from build123d import *

# Parameters (mm, degrees)
BOSS_EXTRUDE1_DEPTH = 3.048
SKETCH2_R           = 1.355900406
CUT_EXTRUDE1_DEPTH  = 430.898988368
SKETCH3_R           = 1.524
CUT_EXTRUDE2_DEPTH  = 430.898988368
CUT_EXTRUDE3_DEPTH  = 430.898988368
BOSS_EXTRUDE2_DEPTH = 3.048
SKETCH5_W           = 73.1256
SKETCH5_H           = 52.8987
SKETCH5_W_2         = 9.017
SKETCH5_H_2         = 13.74935
CUT_EXTRUDE4_DEPTH  = 430.898988368


with BuildPart() as part:
    # Sketch1 → Boss-Extrude1 (new body)
    with BuildSketch(Plane.XY):
        with BuildLine():
            Line((-309.8086, 128.8851), (-305.87795, 128.8851))
            Line((-305.87795, 128.8851), (-301.9473, 132.81575))
            Line((-301.9473, 132.81575), (-301.9473, 150.9704))
            ThreePointArc((-301.9473, 150.9704), (-303.063223164, 153.664476836), (-305.7573, 154.7804))
            Line((-305.7573, 154.7804), (-397.247125, 154.7804))
            ThreePointArc((-397.247125, 154.7804), (-399.946077222, 153.659592612), (-401.0571, 150.956597849))
            Line((-401.0571, 150.956597849), (-401.0571, 148.341))
            Line((-401.0571, 148.341), (-399.1521, 148.341))
            Line((-399.1521, 148.341), (-399.1521, 95.6449))
            Line((-399.1521, 95.6449), (-401.0571, 95.6449))
            Line((-401.0571, 95.6449), (-401.0571, 91.659304166))
            ThreePointArc((-401.0571, 91.659304166), (-399.951018769, 88.947400452), (-397.2472, 87.8217))
            Line((-397.2472, 87.8217), (-378.5565, 87.8217))
            Line((-378.5565, 87.8217), (-368.3165, 91.1883))
            Line((-368.3165, 91.1883), (-315.9973, 91.1883))
            Line((-315.9973, 91.1883), (-305.7573, 87.8217))
            ThreePointArc((-305.7573, 87.8217), (-303.063223164, 88.937623164), (-301.9473, 91.6317))
            Line((-301.9473, 91.6317), (-301.9473, 111.74645))
            Line((-301.9473, 111.74645), (-305.87795, 115.6771))
            Line((-305.87795, 115.6771), (-309.8086, 115.6771))
            Line((-309.8086, 115.6771), (-314.0123, 115.6771))
            Line((-314.0123, 115.6771), (-314.0123, 128.8851))
            Line((-314.0123, 128.8851), (-309.8086, 128.8851))
        make_face()
        Polygon((-395.3675, 92.9525), (-395.3675, 149.2432), (-309.8086, 149.2432), (-309.8086, 132.81575), (-318.2033, 132.81575), (-318.2033, 111.74645), (-309.8086, 111.74645), (-309.8086, 92.9525), align=None, mode=Mode.SUBTRACT)
    extrude(amount=BOSS_EXTRUDE1_DEPTH)

    # Sketch2 → Cut-Extrude1 (cut, through all)
    with BuildSketch(Plane(origin=(0, 0, 0), x_dir=(-1, 0, 0), z_dir=(0, 0, -1))):
        with Locations((305.7573, 150.9704)):
            Circle(SKETCH2_R)
        with Locations((397.247125, 150.9704)):
            Circle(SKETCH2_R)
        with Locations((397.2472, 91.6317)):
            Circle(SKETCH2_R)
        with Locations((305.7573, 91.6317)):
            Circle(SKETCH2_R)
    extrude(amount=-CUT_EXTRUDE1_DEPTH, mode=Mode.SUBTRACT)

    # Sketch3 → Cut-Extrude2 (cut, through all)
    with BuildSketch(Plane(origin=(0, 0, 0), x_dir=(-1, 0, 0), z_dir=(0, 0, -1))):
        with Locations((305.7573, 150.9704)):
            Circle(SKETCH3_R)
        with Locations((397.247125, 150.9704)):
            Circle(SKETCH3_R)
        with Locations((397.2472, 91.6317)):
            Circle(SKETCH3_R)
        with Locations((305.7573, 91.6317)):
            Circle(SKETCH3_R)
    extrude(amount=-CUT_EXTRUDE2_DEPTH, mode=Mode.SUBTRACT)

    # Sketch4 → Cut-Extrude3 (cut, through all)
    with BuildSketch(Plane.XY.offset(3.048)):
        Polygon((-301.9473, 133.57775), (-305.87795, 129.6471), (-314.0123, 129.6471), (-314.0123, 113.6451), (-305.87795, 113.6451), (-301.9473, 109.71445), align=None)
    extrude(amount=-CUT_EXTRUDE3_DEPTH, mode=Mode.SUBTRACT)

    # Sketch4<4> → Boss-Extrude2 (add)
    with BuildSketch(Plane.XY.offset(3.048)):
        Polygon((-318.2033, 111.74645), (-318.2033, 132.81575), (-309.8086, 132.81575), (-309.8086, 149.2432), (-395.3675, 149.2432), (-395.3675, 92.9525), (-309.8086, 92.9525), (-309.8086, 111.74645), align=None)
    extrude(amount=-BOSS_EXTRUDE2_DEPTH)

    # Sketch5 → Cut-Extrude4 (cut, through all)
    with BuildSketch(Plane.XY.offset(3.048)):
        with Locations((-357.6871, 121.98105)):
            Rectangle(SKETCH5_W, SKETCH5_H)
        with Locations((-316.6158, 141.555725)):
            Rectangle(SKETCH5_W_2, SKETCH5_H_2)
        with Locations((-316.6158, 102.406375)):
            Rectangle(SKETCH5_W_2, SKETCH5_H_2)
    extrude(amount=-CUT_EXTRUDE4_DEPTH, mode=Mode.SUBTRACT)


solid = part.part
Verification items for the finished model (mm, model axes). A direction names the side the tool comes from. Coordinates: 2 decimals unless noted, no trailing zeros. Write each loop counter-clockwise with the first axis right and the second up, starting at its lowest first coordinate (ties: lowest second). Pieces come first, ordered by that corner, then holes. Notation, with made-up numbers: M 8,45 L 49,45 A18 cw 49,50 Z; hole C -38.75,3 d6. An arc over 180 degrees is marked long. Use CSV: the item, a comma, the result in double quotes.
Q1. Set-up check for faces 4 (the flat face through (-303.885, 131.64, 1.545)), 5 (the flat face through (-310.95, 89.53, 1.5)), 6 (the flat face through (-317, 134.681, 2)), 7 (the flat face through (-400, 95.645, 2)): record each of +Z, -Z, +X, -X, +Y, -Y from which the full face is reachable in a straight line by a thin tool's end or side.
Computed values:
face 4,"+Z, -Z, +X"
face 5,"+Z, -Z, -Y"
face 6,"+Z, -Z"
face 7,"+Z, -Z, -X"
Q2. Section check C-C, the plane z = 0.7. State how many separate pieces and enclosed holes the cut face has, and give its area (3 significant figures).
Computed values:
separate pieces,"1"
enclosed holes,"5"
area,"1,960 mm²"
Q3. Thickness scan on line 1 along Y through (x, z) = (-317, 1.6); line 2 along Y through (x, z) = (-365, 2); line 3 along X through (y, z) = (105, 0.35). Record the ranges inside material, lowest first. Write a range as [from, to].
Computed values:
line 1,"[91.19, 95.53], [109.28, 134.68], [148.43, 154.78]"
line 2,"[91.19, 95.53], [148.43, 154.78]"
line 3,"[-399.15, -394.25], [-312.11, -301.95]"
Q4. Go/stop test with flat-tipped pins: P1, Ø1.5, axis at y = 144.5, z = 2, coming from the -X side; P2, Ø1.8, axis at x = -397.25, y = 91.63, coming from the +Z side; P3, Ø1, axis at x = -400, z = 1, coming from the -Y side; P4, Ø0.9, axis at x = -311, z = 2, coming from the -Y side. Record where each tip stops, or that it passes through.
Computed values:
P1,"x = -399.15"
P2,"through"
P3,"y = 88.56"
P4,"y = 89.4"
Q5. Mould release check, pull along Y, two halves, no side actions. Record for faces 1 (the flat face through (-352, 92, 0)), 2 (the flat face through (-314.012, 122, 2)), 3 (the flat face through (-373.51, 89.48, 1.5)): pulls with the +Y half, pulls with the -Y half, needs draft (parallel to the pull), parting line crosses it, or undercut.
Computed values:
face 1,"needs draft"
face 2,"undercut"
face 3,"pulls with the -Y half"
Q6. Section check B-B, the plane x = -329.5. Enter the section's corners in (y, z).
Computed values:
outline,"M 91.19,0 L 95.53,0 L 95.53,3.05 L 91.19,3.05 Z; M 148.43,0 L 154.78,0 L 154.78,3.05 L 148.43,3.05 Z"
Q7. Section check A-A, the plane y = 105. Enter the section's corners in (x, z), and give its area (3 significant figures).
Computed values:
outline,"M -399.15,0 L -394.25,0 L -394.25,3.05 L -399.15,3.05 Z; M -312.11,0 L -301.95,0 L -301.95,3.05 L -312.11,3.05 Z"
area,"45.9 mm²"
